Here's how the part is built. I have some questions about the finished solid (model axes, mm). Face numbers are marked on the shaded views. A direction names the side the tool comes from. Round coordinates to 2 decimals unless told otherwise and drop trailing zeros. Order: outer loops, then holes, each group sorted by start corner. A loop starts at its lowest first (then second) coordinate and runs counter-clockwise, first axis right, second up. Notation, with made-up numbers: M 59.5,81.5 L 78.5,81.5 A30 cw 78.5,110.5 Z; hole C 26,-1 d6. An arc over 180 degrees is marked long. Write item = value, one per line. Start each with the question number.
Item 1: We'd pull the mould along Z, two halves only. Please class the marked faces 4, 5 and 6: pulls with the +Z half, pulls with the -Z half, needs draft (parallel to the pull), parting line crosses it, or undercut.
Item 2: I'm going to push flat-ended pins straight in: P1, Ø9.5, axis at x = -7.7, z = 12.5, coming from the +Y side; P2, Ø6, axis at x = 40.5, z = 13.5, coming from the -Y side; P3, Ø7.5, axis at x = 7.7, z = 12.5, coming from the +Y side; P4, Ø10, axis at y = -10.5, z = 17.5, coming from the +X side. Where does each tip first touch, or does it pass through?
Item 3: I want a section at A-A, the plane z = 22. List the corners of the cut face in (x, y) for me, plus the area to 3 significant figures.
Item 4: For the marked faces 1, 2 and 3, which set-ups out of +Z, -Z, +X, -X, +Y, -Y let a thin tool reach every point of the face, with its end or its side?
Item 5: I want a section at B-B, the plane z = 12.5. List the corners of the cut face in (x, y) for me.
Item 6: I want a section at C-C, the plane x = 22. List the corners of the cut face in (y, z) for me, plus the area to 3 significant figures.
Item 7: Please list where these lines run through material, in increasing order: L1, parallel to Y at x = 32, z = 9; L2, parallel to Y at x = 31, z = 8; L3, parallel to Y at x = 3, z = 10.75.
```python
from build123d import *

# Parameters (mm, degrees)
F1_DEPTH = 25
F2_R     = 4.1
F3_DEPTH = 25


with BuildPart() as f1:
    # F0 (on Top) → F1 (new body)
    with BuildSketch(Plane.XY):
        with BuildLine():
            ThreePointArc((-70, 0), (-36.032673, -12.098464), (0, -13.439566))
            Line((0, -13.439566), (30, -19.199381))
            ThreePointArc((30, -19.199381), (44.589191, -16.091), (59.178382, -19.199381))
            ThreePointArc((59.178382, -19.199381), (70.113907, -9.217961), (58.527552, 0))
            ThreePointArc((58.527552, 0), (44.263776, -4.461903), (30, 0))
            Line((30, 0), (0, 0))
            ThreePointArc((0, 0), (-29.481515, -4.146069), (-58.963031, 0))
            Line((-58.963031, 0), (-70, 0))
        make_face()
        with BuildLine():
            ThreePointArc((57.279562, -5.566995), (62.605872, -5.005802), (65.444396, -9.54753))
            ThreePointArc((65.444396, -9.54753), (62.605872, -14.089259), (57.279562, -13.528066))
            Line((57.279562, -13.528066), (30, -9.59969))
            Line((30, -9.59969), (57.279562, -5.566995))
        make_face(mode=Mode.SUBTRACT)
    extrude(amount=F1_DEPTH)

    # F2 (on face) → F3 (cut)
    with BuildSketch(Plane(origin=(0, 0, 0), x_dir=(-1, 0, 0), z_dir=(0, 1, 0))):
        with Locations((-7.695812, 12.5)):
            Circle(F2_R)
        with Locations((7.695812, 12.5)):
            Circle(F2_R)
        with Locations((32.304188, 12.5)):
            Circle(F2_R)
        with Locations((47.695812, 12.5)):
            Circle(F2_R)
    extrude(amount=-F3_DEPTH, mode=Mode.SUBTRACT)


solid = f1.part
```
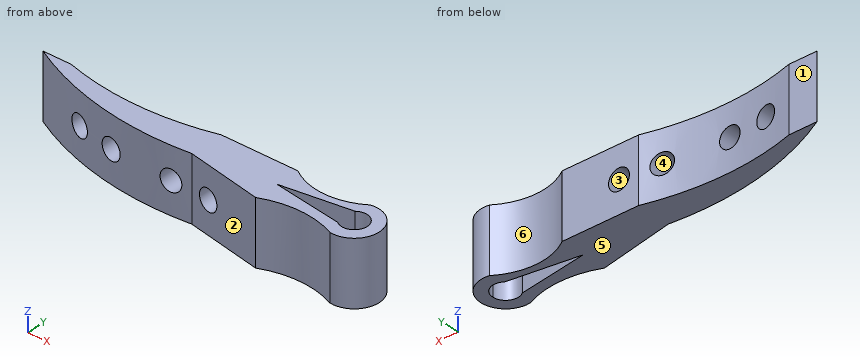
Filled in:
q1.face_4 = undercut
q1.face_5 = pulls with the -Z half
q1.face_6 = needs draft
q2.P1 = -0.8
q2.P2 = -16.8
q2.P3 = through
q2.P4 = 70.12
q3.outline = M -70,0 A118.69 ccw 0,-13.44 L 30,-19.2 A35.79 cw 59.18,-19.2 A9.73 ccw long 58.53,0 A25.03 cw 30,0 L 0,0 A106.89 cw -58.96,0 Z; hole M 30,-9.6 L 57.28,-13.53 A5.05 ccw 65.44,-9.55 A5.05 ccw 57.28,-5.57 Z
q3.area = 1,460 mm^2
q4.face_1 = +Z, -Z, -X, +Y
q4.face_2 = +Z, -Z, -Y
q4.face_3 = +Y, -Y
q5.outline = M -70,0 A118.69 ccw -51.8,-7.93 L -51.8,-1.79 A106.89 cw -58.96,0 Z; M -43.6,-10.39 A118.69 ccw -36.4,-12.03 L -36.4,-3.92 A106.89 cw -43.6,-3.21 Z; M -28.2,-13.33 A118.69 ccw -11.8,-14.21 L -11.8,-2.67 A106.89 cw -28.2,-4.14 Z; M -3.6,-13.8 A118.69 ccw 0,-13.44 L 3.6,-14.13 L 3.6,0 L 0,0 A106.89 cw -3.6,-0.96 Z; M 11.8,-15.7 L 30,-19.2 A35.79 cw 59.18,-19.2 A9.73 ccw long 58.53,0 A25.03 cw 30,0 L 11.8,0 Z; hole M 30,-9.6 L 57.28,-13.53 A5.05 ccw 65.44,-9.55 A5.05 ccw 57.28,-5.57 Z
q6.outline = M -17.66,0 L 0,0 L 0,25 L -17.66,25 Z
q6.area = 442 mm^2
q7.L1 = -18.38 to -9.89, -9.3 to -1.25
q7.L2 = -18.77 to -9.74, -9.45 to -0.66
q7.L3 = -14.02 to 0
